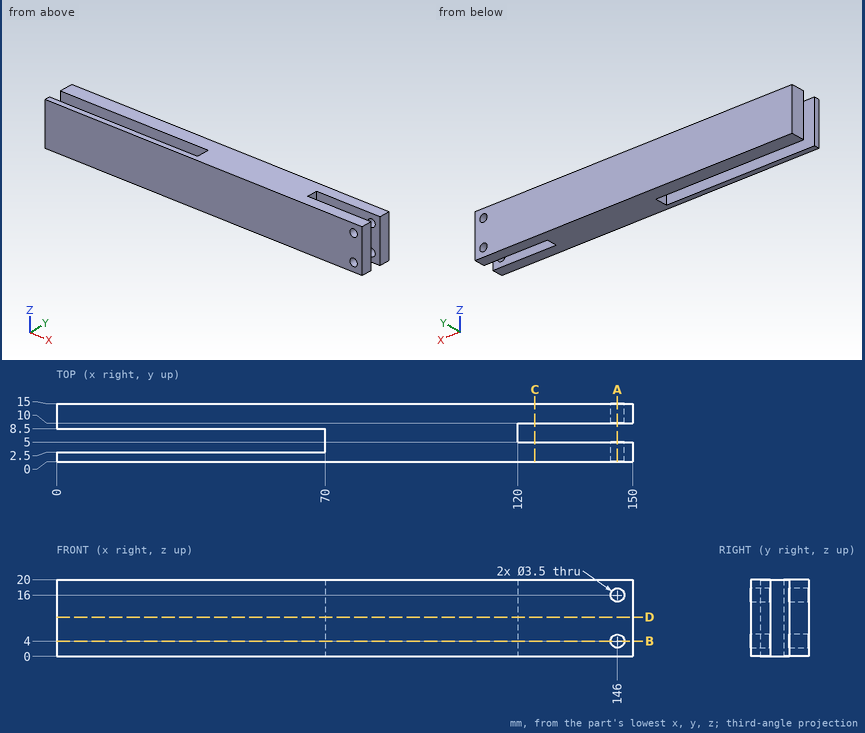
Part print with two shaded views. Sizes in mm from the minimum x, y, z corner. Coordinates: 2 decimals unless noted, no trailing zeros. Order: outer loops, then holes, each group sorted by start corner. A loop starts at its lowest first (then second) coordinate and runs counter-clockwise, first axis right, second up.
(1) Saw through at C-C, the plane x = 124.5. Write the cut outline in (y, z).
Solution:
outline: (0, 0) - (5, 0) - (5, 20) - (0, 20) - close; (10, 0) - (15, 0) - (15, 20) - (10, 20) - close
(2) Pin check, flat tips, straight feed: pin 1 Ø2 at (x, z) = (146, 16) entering from -Y; pin 2 Ø1.5 at (y, z) = (8.5, 12.5) entering from +X; pin 3 Ø1 at (y, z) = (3.5, 10) entering from -X. Stop position of each tip, or through.
Solution:
pin 1: passes through
pin 2: stops at x = 120
pin 3: stops at x = 70
(3) Saw through at A-A, the plane x = 146. Write the cut outline in (y, z), and give its area (3 significant figures).
Solution:
outline: (0, 0) - (5, 0) - (5, 2.25) - (0, 2.25) - close; (0, 5.75) - (5, 5.75) - (5, 14.25) - (0, 14.25) - close; (0, 17.75) - (5, 17.75) - (5, 20) - (0, 20) - close; (10, 0) - (15, 0) - (15, 2.25) - (10, 2.25) - close; (10, 5.75) - (15, 5.75) - (15, 14.25) - (10, 14.25) - close; (10, 17.75) - (15, 17.75) - (15, 20) - (10, 20) - close
area: 130 mm2
(4) Drill centre lines: L1, parallel to Z at x = 146, y = 1.6; L2, parallel to X at y = 12.45, z = 16; L3, parallel to Y at x = 120.5, z = 5.25. Where is each one in solid material? Low to high.
Solution:
L1: z = 0 to 2.25, 5.75 to 14.25, 17.75 to 20
L2: x = 0 to 144.25, 147.75 to 150
L3: y = 0 to 5, 10 to 15
(5) Saw through at D-D, the plane z = 10.25. Write the cut outline in (x, y), and give its area (3 significant figures).
Solution:
outline: (0, 0) - (150, 0) - (150, 5) - (120, 5) - (120, 10) - (150, 10) - (150, 15) - (0, 15) - (0, 8.5) - (70, 8.5) - (70, 2.5) - (0, 2.5) - close
area: 1,680 mm2
(6) Saw through at B-B, the plane z = 4. Write the cut outline in (x, y).
Solution:
outline: (0, 0) - (144.25, 0) - (144.25, 5) - (120, 5) - (120, 10) - (144.25, 10) - (144.25, 15) - (0, 15) - (0, 8.5) - (70, 8.5) - (70, 2.5) - (0, 2.5) - close; (147.75, 0) - (150, 0) - (150, 5) - (147.75, 5) - close; (147.75, 10) - (150, 10) - (150, 15) - (147.75, 15) - close
